from build123d import *

# Parameters (mm, degrees)
POCKET_DEPTH = 2


with BuildPart() as part:
    # Sketch → Revolution (revolve)
    with BuildSketch(Plane.XY):
        with BuildLine():
            Line((2, 0), (3.5, 0))
            Line((3.5, 0), (3.5, -3.6))
            ThreePointArc((3.1, -4), (3.382843, -3.882843), (3.5, -3.6))
            Line((3.1, -4), (0, -4))
            Line((0, -4), (0, 12))
            Line((0, 12), (1.57, 12))
            Line((1.57, 12), (2, 11.751739))
            Line((2, 11.751739), (2, 0))
        make_face()
    revolve(axis=Axis((0, 0, 0), (0, 1, 0)))

    # Sketch001 → Pocket (cut)
    with BuildSketch(Plane.XZ.offset(4)):
        Polygon((-1.5, 0.866025), (-1.5, -0.866025), (0, -1.732051), (1.5, -0.866025), (1.5, 0.866025), (0, 1.732051), align=None)
    extrude(amount=-POCKET_DEPTH, mode=Mode.SUBTRACT)


solid = part.part
Model file for the job. Use its own axes, mm. A direction names the side the tool comes from. Coordinates: 2 decimals unless noted, no trailing zeros. Write each loop counter-clockwise with the first axis right and the second up, starting at its lowest first coordinate (ties: lowest second). Pieces come first, ordered by that corner, then holes. Notation, with made-up numbers: (81.25, 38.5) -> (92.25, 38.5) arc R20 ccw to (92.25, 45.5) -> close; hole circle Ø4 at (13.5, 82). An arc over 180 degrees is marked (long way). One line per item, written item: value. Start each with the question number.
1) Probe probe 1 along Z at (x, y) = (-1, 10.5); probe 2 along X at (y, z) = (-3, 1.25). List the from-to ranges inside material, lowest first.
2) Slice it at B-B on y = -1.5. Write the cut outline in (x, z).
3) Slice it at A-A on z = 0. Write the cut outline in (x, y), then the cut area to 3 significant figures.
4) Which spindle directions (+Z, -Z, +X, -X, +Y, -Y) get a long thin tool onto all of the face, cutting with end or side? Do faces 5 (the face through (0.74, -3.014, -1.305)), 6 (the face through (3.233, -1.825, 1.341)). Say none if no direction does.
5) Pull direction X, two halves, no side cores. Call faces 1 (the face through (-0.76, -3.014, -1.293)), 2 (the face through (0, 6, 2)), 3 (the face through (-2, 0, 2)), 4 (the face through (0, -2, 0)): +X half, -X half, draft (parallel to the pull), parting line (faces both ways), or undercut.
6) Flat gauge pins, fed straight in: pin 1 Ø1.5 at (x, y) = (-1.5, 1) entering from +Z; pin 2 Ø0.9 at (y, z) = (-2.5, -0.5) entering from +X; pin 3 Ø1 at (x, z) = (-1.5, -2.5) entering from +Y; pin 4 Ø2 at (y, z) = (8, -2) entering from -X. Where does each tip first touch, or does it go through?
Answers follow:
1. probe 1: -1.73 to 1.73
1. probe 2: -3.27 to -0.83, 0.83 to 3.27
2. outline: circle Ø7 at (0, 0)
3. outline: (-3.5, -3.6) arc R0.4 ccw to (-3.1, -4) -> (-1.5, -4) -> (-1.5, -2) -> (1.5, -2) -> (1.5, -4) -> (3.1, -4) arc R0.4 ccw to (3.5, -3.6) -> (3.5, 0) -> (2, 0) -> (2, 11.75) -> (1.57, 12) -> (-1.57, 12) -> (-2, 11.75) -> (-2, 0) -> (-3.5, 0) -> close
3. area: 69.8 mm2
4. face 5: -Y
4. face 6: +Y, -Y
5. face 1: undercut
5. face 2: parting line
5. face 3: draft
5. face 4: undercut
6. pin 1: z = 1.85
6. pin 2: x = 3.5
6. pin 3: y = 0
6. pin 4: x = -1.73
